Build history of the part. All positions in model axes, mm. A direction names the side the tool comes from. Coordinates: 2 decimals unless noted, no trailing zeros. Loops run counter-clockwise (first coordinate to the right, second up) from the corner with the lowest first, then second, coordinate; pieces in that order, holes last. Notation, with made-up numbers: (-3.5, -7.5) - (19.5, -7.5) arc R7 cw to (19.5, 4.5) - close; hole circle Ø2 at (48.25, 28). An arc over 180 degrees is marked (long way). One line per item, written item: value.
```python
from build123d import *

# Parameters (mm, degrees)
F0_W     = 25.4
F0_H     = 38.1
F1_DEPTH = 6.35
F2_W     = 18.8976
F2_H     = 31.5976
F3_DEPTH = 3.175
F4_R     = 3.3782
F5_DEPTH = 25.4


with BuildPart() as f1:
    # F0 (on Front) → F1 (new body)
    with BuildSketch(Plane.XZ):
        with Locations((12.7, 19.05)):
            Rectangle(F0_W, F0_H)
    extrude(amount=-F1_DEPTH)

    # F2 (on face) → F3 (join)
    with BuildSketch(Plane.XZ):
        with Locations((12.7, 19.05)):
            Rectangle(F2_W, F2_H)
    extrude(amount=F3_DEPTH)

    # F4 (on face) → F5 (cut)
    with BuildSketch(Plane.XZ.offset(3.175)):
        with Locations((12.7, 19.05)):
            Circle(F4_R)
    extrude(amount=-F5_DEPTH, mode=Mode.SUBTRACT)


solid = f1.part
```
Item 1: Cut at B-B, the plane z = 19.05. Write the cut outline in (x, y) (3 decimals), then the cut area to 3 significant figures.
Check result:
outline: (0, 0) - (3.251, 0) - (3.251, -3.175) - (9.322, -3.175) - (9.322, 6.35) - (0, 6.35) - close; (16.078, -3.175) - (22.149, -3.175) - (22.149, 0) - (25.4, 0) - (25.4, 6.35) - (16.078, 6.35) - close
area: 157 mm^2
Item 2: Pull direction Z, two halves, no side cores. Call faces 1 (the face through (13, 3, 38.1)), 2 (the face through (11.97, 1.52, 15.75)), 3 (the face through (22.149, -2, 19)): released by +Z, released by -Z, zero draft, split by the parting line, or undercut.
Check result:
face 1: released by +Z
face 2: undercut
face 3: zero draft
Item 3: Cut at A-A, the plane x = 12.7. Write the cut outline in (y, z) (3 decimals), then the cut area to 3 significant figures.
Check result:
outline: (-3.175, 3.251) - (0, 3.251) - (0, 0) - (6.35, 0) - (6.35, 15.672) - (-3.175, 15.672) - close; (-3.175, 22.428) - (6.35, 22.428) - (6.35, 38.1) - (0, 38.1) - (0, 34.849) - (-3.175, 34.849) - close
area: 278 mm^2
Item 4: Drop flat-ended pins along their axis: P1, Ø8, axis at x = 12.7, z = 19.05, coming from the +Y side; P2, Ø1.6, axis at y = -1.5, z = 20, coming from the -X side; P3, Ø2.5, axis at y = -2, z = 25, coming from the +X side; P4, Ø3.5, axis at x = 16.5, y = -2.5, coming from the +Z side. Give the stop position or say it passes through.
Check result:
P1: stops at y = 6.35
P2: stops at x = 3.25
P3: stops at x = 22.15
P4: stops at z = 34.85
Item 5: Probe probe 1 along Z at (x, y) = (12.7, 2); probe 2 along Z at (x, y) = (12.5, -1.5); probe 3 along X at (y, z) = (5.25, 22). List the from-to ranges inside material, lowest first. Write a range as from..to.
Check result:
probe 1: z = 0..15.67, 22.43..38.1
probe 2: z = 3.25..15.68, 22.42..34.85
probe 3: x = 0..11.05, 14.35..25.4
Item 6: Cut at D-D, the plane x = 8. Write the cut outline in (y, z) (3 decimals), then the cut area to 3 significant figures.
Check result:
outline: (-3.175, 3.251) - (0, 3.251) - (0, 0) - (6.35, 0) - (6.35, 38.1) - (0, 38.1) - (0, 34.849) - (-3.175, 34.849) - close
area: 342 mm^2
Item 7: Tool access for faces 4 (the face through (3.251, -2, 19)), 5 (the face through (13, -2, 34.849)), 6 (the face through (13, -2, 3.251)), 7 (the face through (13, 6.35, 24)): list every direction of +Z, -Z, +X, -X, +Y, -Y with a clear straight run to the whole face (end or side of a thin tool).
Check result:
face 4: +Z, -Z, -X, -Y
face 5: +Z, +X, -X, -Y
face 6: -Z, +X, -X, -Y
face 7: +Z, -Z, +X, -X, +Y
Item 8: Cut at C-C, the plane y = -0.75. Write the cut outline in (x, z), then the cut area to 3 significant figures.
Check result:
outline: (3.25, 3.25) - (22.15, 3.25) - (22.15, 34.85) - (3.25, 34.85) - close; hole circle Ø6.76 at (12.7, 19.05)
area: 561 mm^2
